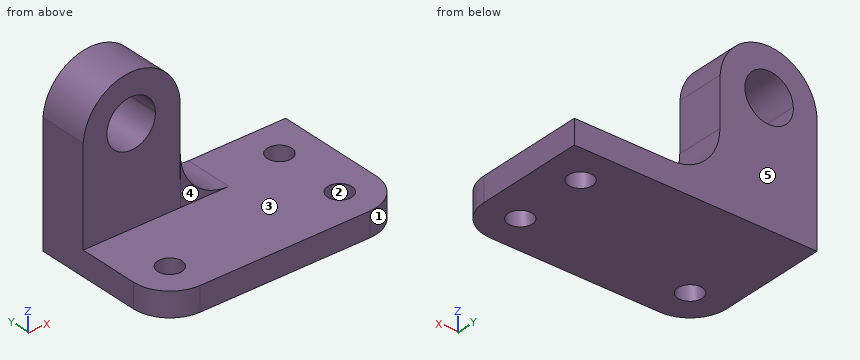
from build123d import *

# Parameters (mm, degrees)
F0_W     = 63.5
F0_H     = 38.1
F1_DEPTH = 6.35
F2_R     = 3.175
F3_DEPTH = 6.35
F4_W     = 38.1
F4_H     = 12.7
F5_DEPTH = 38.1
F7_DEPTH = 25.4


with BuildPart() as f1:
    # F0 (on Top) → F1 (new body)
    with BuildSketch(Plane.XY):
        with Locations((-8.3569418639, 1.878844718)):
            Rectangle(F0_W, F0_H)
    extrude(amount=F1_DEPTH)

    # F2 (on face) → F3 (cut)
    with BuildSketch(Plane.XY.offset(6.35)):
        with Locations((-30.5819418639, -7.646155282)):
            Circle(F2_R)
        with Locations((13.8680581361, -7.646155282)):
            Circle(F2_R)
        with Locations((13.8680581361, 11.403844718)):
            Circle(F2_R)
        with BuildLine():
            ThreePointArc((-30.5819418639, -17.171155282), (-37.3117803251, -14.3759937432), (-40.1069418639, -7.646155282))
            Line((-40.1069418639, -7.646155282), (-40.1069418639, -17.171155282))
            Line((-40.1069418639, -17.171155282), (-30.5819418639, -17.171155282))
        make_face()
        with BuildLine():
            ThreePointArc((23.3930581361, -7.646155282), (20.5978084208, -14.3759055667), (13.8680581361, -17.171155282))
            Line((13.8680581361, -17.171155282), (23.3930581361, -17.171155282))
            Line((23.3930581361, -17.171155282), (23.3930581361, -7.646155282))
        make_face()
    extrude(amount=-F3_DEPTH, mode=Mode.SUBTRACT)

    # F4 (on face) → F5 (join)
    with BuildSketch(Plane.XY.offset(6.35)):
        with Locations((-21.0569418639, 14.578844718)):
            Rectangle(F4_W, F4_H)
    extrude(amount=F5_DEPTH)

    # F6 (on face) → F7 (cut)
    with BuildSketch(Plane.XZ.offset(-8.228844718)):
        with BuildLine():
            Line((-33.9147208913, 31.75), (-21.2317441048, 31.75))
            ThreePointArc((-21.2317441048, 31.75), (-27.573232498, 37.771328495), (-33.9147208913, 31.75))
        make_face()
        with BuildLine():
            ThreePointArc((-21.223232498, 31.421328495), (-21.2253607564, 31.5857193445), (-21.2317441048, 31.75))
            Line((-21.2317441048, 31.75), (-33.9147208913, 31.75))
            ThreePointArc((-33.9147208913, 31.75), (-27.7376233476, 25.0734567533), (-21.223232498, 31.421328495))
        make_face()
        with BuildLine():
            Line((-14.7069418639, 6.35), (-14.7069418639, 19.05))
            ThreePointArc((-14.7069418639, 19.05), (-10.987197985, 10.0697438789), (-2.0069418639, 6.35))
            Line((-2.0069418639, 6.35), (-2.0069418639, 31.75))
            Line((-2.0069418639, 31.75), (-14.7562308182, 31.75))
            Line((-14.7562308182, 31.75), (-14.7069418639, 6.35))
        make_face()
        Polygon((-14.7808752954, 44.45), (-14.7562308182, 31.75), (-2.0069418639, 31.75), (-2.0069418639, 44.45), align=None)
        with BuildLine():
            ThreePointArc((-40.1069418639, 31.75), (-27.4315863411, 43.6414101491), (-14.7562308182, 31.75))
            Line((-14.7562308182, 31.75), (-14.7808752954, 44.45))
            Line((-14.7808752954, 44.45), (-40.1069418639, 44.45))
            Line((-40.1069418639, 44.45), (-40.1069418639, 31.75))
        make_face()
    extrude(amount=-F7_DEPTH, mode=Mode.SUBTRACT)


solid = f1.part
The model under review builds one solid part; all positions refer to its coordinate system, in mm. Face numbers are marked on the shaded views. A direction names the side the tool comes from. Round coordinates to 2 decimals unless told otherwise and drop trailing zeros. Loops run counter-clockwise (first coordinate to the right, second up) from the corner with the lowest first, then second, coordinate; pieces in that order, holes last. Notation, with made-up numbers: M 25.25,5.25 L 31.25,5.25 A25 ccw 31.25,28.25 Z; hole C 33.25,-7.75 d2. An arc over 180 degrees is marked long. Answer as CSV lines item,"result". Start each with the question number.
Item 1: Consider section C-C (z = 36). Write out the cut boundary in (x, y), then the cut area to 3 significant figures.
Item 2: Insertion check: P1, Ø7.5, axis at x = -27.5, z = 24.5, coming from the -Y side; P2, Ø6, axis at x = 6, y = -2, coming from the -Z side; P3, Ø8, axis at x = 2.5, y = 15.5, coming from the +Z side; P4, Ø4, axis at x = 13.87, y = 11.4, coming from the -Z side. Each pin has a flat end and moves straight along its axis. Give the tip position at first contact, or say it passes through.
Item 3: Mouldability with a two-part tool opening along Y and no side actions: class the marked faces 1, 2 and 3 as released by +Y, released by -Y, zero draft, split by the parting line, or undercut.
Item 4: Consider section A-A (y = 13). Write out the cut boundary in (x, z), then the cut area to 3 significant figures.
Item 5: Wall thickness on line 1 (X direction, y = 10, z = 25); line 2 (Y direction, x = -24, z = 19); line 3 (Z direction, x = -28.5, y = 13): over which ranges is each line inside the solid? List them lowest first. Write a range as [from, to].
Item 6: Consider section B-B (x = -25). Write out the cut boundary in (y, z), then the cut area to 3 significant figures.
Item 7: For the marked faces 4 and 5, list the 3-axis set-ups (+Z, -Z, +X, -X, +Y, -Y) from which the entire face can be reached by the end or side of a thin tool; tool diameter is ignored.
Item 8: Consider section D-D (x = -31.5). Write out the cut boundary in (y, z), then the cut area to 3 significant figures.
Answer:
1,outline,"M -39.08,8.23 L -31.97,8.23 L -31.97,20.93 L -39.08,20.93 Z; M -23.17,8.23 L -15.78,8.23 L -15.78,20.93 L -23.17,20.93 Z"
1,area,"184 mm^2"
2,P1,"stops at y = 8.23"
2,P2,"stops at z = 0"
2,P3,"stops at z = 6.35"
2,P4,"passes through"
3,face 1,"released by -Y"
3,face 2,"undercut"
3,face 3,"zero draft"
4,outline,"M -40.11,0 L 11.12,0 L 11.12,6.35 L -2.01,6.35 A12.7 cw -14.71,19.05 L -14.71,6.35 L -14.76,31.75 A12.7 ccw -40.11,31.75 Z; M 16.61,0 L 23.39,0 L 23.39,6.35 L 16.61,6.35 Z; hole C -27.57,31.42 d12.7"
4,area,"1,150 mm^2"
5,line 1,"x = [-40.11, -14.74]"
5,line 2,"y = [8.23, 20.93]"
5,line 3,"z = [0, 25.14], [37.7, 43.6]"
6,outline,"M -17.17,0 L 20.93,0 L 20.93,25.62 L 8.23,25.62 L 8.23,6.35 L -17.17,6.35 Z; M 8.23,37.23 L 20.93,37.23 L 20.93,43.41 L 8.23,43.41 Z"
6,area,"565 mm^2"
7,face 4,"+Z, +X, -X, -Y"
7,face 5,"+Z, -Z, +X, -X, +Y"
8,outline,"M -17.13,0 L -10.69,0 L -10.69,6.35 L -17.13,6.35 Z; M -4.61,0 L 20.93,0 L 20.93,26.43 L 8.23,26.43 L 8.23,6.35 L -4.61,6.35 Z; M 8.23,36.41 L 20.93,36.41 L 20.93,42.97 L 8.23,42.97 Z"
8,area,"541 mm^2"
